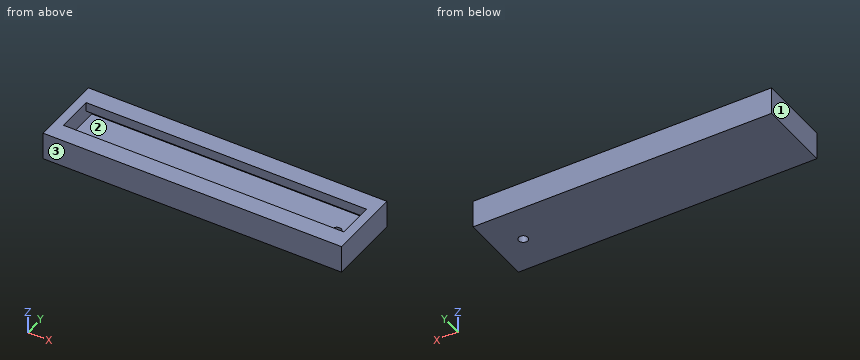
from build123d import *

# Parameters (mm, degrees)
SKETCH1_W           = 65
SKETCH1_H           = 16
BOSS_EXTRUDE1_DEPTH = 2
SKETCH2_W           = 65
SKETCH2_H           = 16
SKETCH2_W_2         = 61
SKETCH2_H_2         = 12
BOSS_EXTRUDE2_DEPTH = 2
SKETCH4_W           = 65
SKETCH4_H           = 16
SKETCH4_W_2         = 61
SKETCH4_H_2         = 8
BOSS_EXTRUDE3_DEPTH = 2
SKETCH6_R           = 1
CUT_EXTRUDE2_DEPTH  = 34.708307581


with BuildPart() as part:
    # Sketch1 → Boss-Extrude1 (new body)
    with BuildSketch(Plane.XY):
        Rectangle(SKETCH1_W, SKETCH1_H)
    extrude(amount=BOSS_EXTRUDE1_DEPTH)

    # Sketch2 → Boss-Extrude2 (add)
    with BuildSketch(Plane.XY.offset(2)):
        Rectangle(SKETCH2_W, SKETCH2_H)
        Rectangle(SKETCH2_W_2, SKETCH2_H_2, mode=Mode.SUBTRACT)
    extrude(amount=BOSS_EXTRUDE2_DEPTH)

    # Sketch4 → Boss-Extrude3 (add)
    with BuildSketch(Plane.XY.offset(4)):
        Rectangle(SKETCH4_W, SKETCH4_H)
        Rectangle(SKETCH4_W_2, SKETCH4_H_2, mode=Mode.SUBTRACT)
    extrude(amount=BOSS_EXTRUDE3_DEPTH)

    # Sketch6 → Cut-Extrude2 (cut, through all)
    with BuildSketch(Plane.XY.offset(2)):
        with Locations((26.5, 0)):
            Circle(SKETCH6_R)
    extrude(amount=-CUT_EXTRUDE2_DEPTH, mode=Mode.SUBTRACT)


solid = part.part
CAD build for the part. Positions are in the model's coordinates, mm. Face numbers are marked on the shaded views. Round coordinates to 2 decimals unless told otherwise and drop trailing zeros. Loops run counter-clockwise (first coordinate to the right, second up) from the corner with the lowest first, then second, coordinate; pieces in that order, holes last.
(1) Cut at B-B (x = 26.5). Give the cut face in (y, z).
(2) Drop a flat-ended pin along its axis: pin 1 (3.5 mm diameter, centred on x = 5.5, y = 0, fed in from +Z). Give the stop position or say it passes through.
(3) Two-plate mould, pull along Y, no slides. Class the marked faces 1, 2 and 3: +Y half, -Y half, draft (parallel to the pull), parting line (faces both ways), or undercut.
(4) Cut at D-D (x = -20). Give the cut face in (y, z).
(5) Cut at A-A (y = 0). Give the cut face in (x, z).
(6) Cut at C-C (z = 3.2). Give the cut face in (x, y).
(7) Wall check: line 1 along Y through (x, z) = (-29, 2.45); line 2 along Y through (x, z) = (26.5, 1.05); line 3 along Z through (x, y) = (20, -5.5). Give the ranges that are in metal, low to high.
Findings below:
1. outline: (-8, 0) - (-1, 0) - (-1, 2) - (-6, 2) - (-6, 4) - (-4, 4) - (-4, 6) - (-8, 6) - close; (1, 0) - (8, 0) - (8, 6) - (4, 6) - (4, 4) - (6, 4) - (6, 2) - (1, 2) - close
2. pin 1: stops at z = 2
3. face 1: draft
3. face 2: undercut
3. face 3: -Y half
4. outline: (-8, 0) - (8, 0) - (8, 6) - (4, 6) - (4, 4) - (6, 4) - (6, 2) - (-6, 2) - (-6, 4) - (-4, 4) - (-4, 6) - (-8, 6) - close
5. outline: (-32.5, 0) - (25.5, 0) - (25.5, 2) - (-30.5, 2) - (-30.5, 6) - (-32.5, 6) - close; (27.5, 0) - (32.5, 0) - (32.5, 6) - (30.5, 6) - (30.5, 2) - (27.5, 2) - close
6. outline: (-32.5, -8) - (32.5, -8) - (32.5, 8) - (-32.5, 8) - close; hole (-30.5, -6) - (30.5, -6) - (30.5, 6) - (-30.5, 6) - close
7. line 1: y = -8 to -6, 6 to 8
7. line 2: y = -8 to -1, 1 to 8
7. line 3: z = 0 to 2, 4 to 6
